Work out the finished part from the listing and answer in its coordinate system (mm). A direction names the side the tool comes from. Give positions to 0.01 mm unless a question says otherwise; leave off trailing zeros. Order: outer loops, then holes, each group sorted by start corner. A loop starts at its lowest first (then second) coordinate and runs counter-clockwise, first axis right, second up. Notation, with made-up numbers: (69, 39) - (106, 39) arc R18 cw to (106, 51) - close; hole circle Ø10 at (77.5, 59.5). An arc over 180 degrees is marked (long way). Return JSON: item names as keys, results as strings. Group by question number.
from build123d import *

# Parameters (mm, degrees)
SKETCH1_W                      = 57.15
SKETCH1_H                      = 32.639
BOSS_EXTRUDE1_DEPTH            = 0.762
F_3_0MM_DOWEL_HOLE1_D          = 3
SKETCH5_W                      = 4.5
SKETCH5_H                      = 5.9
BOSS_EXTRUDE2_DEPTH            = 6
SKETCH6_W                      = 3.23
SKETCH6_H                      = 4.63
CUT_EXTRUDE1_DEPTH             = 5.08
SKETCH7_R                      = 0.25
BOSS_EXTRUDE3_DEPTH            = 3.4
BOSS_EXTRUDE4_DEPTH            = 22.86
F_1_5MM_DOWEL_HOLE1_AT_2_COUNT = 2
F_1_5MM_DOWEL_HOLE1_AT_2_PITCH = 2.286
F_1_5MM_DOWEL_HOLE1_AT_3_COUNT = 2
F_1_5MM_DOWEL_HOLE1_AT_3_PITCH = 4.572
F_1_5MM_DOWEL_HOLE1_AT_4_COUNT = 2
F_1_5MM_DOWEL_HOLE1_AT_4_PITCH = 6.858
F_1_5MM_DOWEL_HOLE1_AT_5_COUNT = 2
F_1_5MM_DOWEL_HOLE1_AT_5_PITCH = 9.144
F_1_5MM_DOWEL_HOLE1_AT_6_COUNT = 2
F_1_5MM_DOWEL_HOLE1_AT_6_PITCH = 11.43
F_1_5MM_DOWEL_HOLE1_AT_7_COUNT = 2
F_1_5MM_DOWEL_HOLE1_AT_7_PITCH = 13.716
F_1_5MM_DOWEL_HOLE1_AT_8_COUNT = 2
F_1_5MM_DOWEL_HOLE1_AT_8_PITCH = 16.002
F_1_5MM_DOWEL_HOLE1_AT_9_COUNT = 2
F_1_5MM_DOWEL_HOLE1_AT_9_PITCH = 18.288
SKETCH13_W                     = 1.016
SKETCH13_H                     = 2.54
CUT_EXTRUDE2_DEPTH             = 1.27
LPATTERN1_COUNT                = 9
LPATTERN1_PITCH                = 2.286
MIRROR1_COPY_9_SKETCH_W        = 1.016
MIRROR1_COPY_9_SKETCH_H        = 2.54
MIRROR1_COPY_9_DEPTH           = 1.27
MIRROR1_COPY_10_SKETCH_W       = 1.016
MIRROR1_COPY_10_SKETCH_H       = 2.54
MIRROR1_COPY_10_DEPTH          = 1.27
MIRROR1_COPY_11_SKETCH_W       = 1.016
MIRROR1_COPY_11_SKETCH_H       = 2.54
MIRROR1_COPY_11_DEPTH          = 1.27
MIRROR1_COPY_12_SKETCH_W       = 1.016
MIRROR1_COPY_12_SKETCH_H       = 2.54
MIRROR1_COPY_12_DEPTH          = 1.27
MIRROR1_COPY_13_SKETCH_W       = 1.016
MIRROR1_COPY_13_SKETCH_H       = 2.54
MIRROR1_COPY_13_DEPTH          = 1.27
MIRROR1_COPY_14_SKETCH_W       = 1.016
MIRROR1_COPY_14_SKETCH_H       = 2.54
MIRROR1_COPY_14_DEPTH          = 1.27
MIRROR1_COPY_15_SKETCH_W       = 1.016
MIRROR1_COPY_15_SKETCH_H       = 2.54
MIRROR1_COPY_15_DEPTH          = 1.27
MIRROR1_COPY_16_SKETCH_W       = 1.016
MIRROR1_COPY_16_SKETCH_H       = 2.54
MIRROR1_COPY_16_DEPTH          = 1.27
SKETCH15_R                     = 5.715
BOSS_EXTRUDE5_DEPTH            = 9.652
SKETCH16_R                     = 1.905
CUT_EXTRUDE3_DEPTH             = 2.54


with BuildPart() as part:
    # Sketch1 → Boss-Extrude1 (new body)
    with BuildSketch(Plane(origin=(0, 0, 0), x_dir=(1, 0, 0), z_dir=(0, 1, 0))):
        Rectangle(SKETCH1_W, SKETCH1_H)
    extrude(amount=BOSS_EXTRUDE1_DEPTH)

    # Ø3.0mm Dowel Hole1 (through all)
    with Locations(Plane(origin=(0, 0.762, 0), x_dir=(1, 0, 0), z_dir=(0, 1, 0))):
        with Locations((-25.4, 13.1445), (-25.4, -13.1445), (25.4, -13.1445), (25.4, 13.1445)):
            Hole(F_3_0MM_DOWEL_HOLE1_D / 2)

    # Sketch5 → Boss-Extrude2 (add)
    with BuildSketch(Plane(origin=(0, 0.762, 0), x_dir=(1, 0, 0), z_dir=(0, 1, 0))):
        with Locations((-26.325, 0)):
            Rectangle(SKETCH5_W, SKETCH5_H)
    extrude(amount=BOSS_EXTRUDE2_DEPTH)

    # Sketch6 → Cut-Extrude1 (cut)
    with BuildSketch(Plane(origin=(0, 6.762, 0), x_dir=(1, 0, 0), z_dir=(0, 1, 0))):
        with Locations((-26.325, 0)):
            Rectangle(SKETCH6_W, SKETCH6_H)
    extrude(amount=-CUT_EXTRUDE1_DEPTH, mode=Mode.SUBTRACT)

    # Sketch7 → Boss-Extrude3 (add)
    with BuildSketch(Plane(origin=(0, 1.682, 0), x_dir=(1, 0, 0), z_dir=(0, 1, 0))):
        with Locations(Location((-26.875, 1, 0), (0, 0, 270))):
            Circle(SKETCH7_R)
        with Locations(Location((-26.875, -1, 0), (0, 0, 270))):
            Circle(SKETCH7_R)
    extrude(amount=BOSS_EXTRUDE3_DEPTH)

    # Sketch9 → Boss-Extrude4 (add)
    with BuildSketch(Plane(origin=(-24.075, 0, 0), x_dir=(0, 0, -1), z_dir=(1, 0, 0))):
        Polygon((0, 0), (0, 6.35), (2.54, 6.35), (3.926726593, 10.16), (7.736726593, 10.16), (8.89, 6.35), (8.89, 0), align=None)
    boss_extrude4 = extrude(amount=BOSS_EXTRUDE4_DEPTH)

    # Sketch11 → Ø1.5mm Dowel Hole1 (revolve, cut)
    with BuildSketch(Plane(origin=(-21.789, 10.16, -5.831726593), x_dir=(0, 0, 1), z_dir=(1, 0, 0))):
        Polygon((0, 0), (0, 0.704645464), (0.75, 0.254), (0.75, 0), align=None)
    f_1_5mm_dowel_hole1 = revolve(axis=Axis((-21.789, 16.51, -5.831726593), (0, -1, 0)), mode=Mode.SUBTRACT)

    # Ø1.5mm Dowel Hole1 at 2: Ø1.5mm Dowel Hole1 ×2
    with Locations(*[(i * F_1_5MM_DOWEL_HOLE1_AT_2_PITCH, 0, 0) for i in range(1, F_1_5MM_DOWEL_HOLE1_AT_2_COUNT)]):
        add(f_1_5mm_dowel_hole1, mode=Mode.SUBTRACT)

    # Ø1.5mm Dowel Hole1 at 3: Ø1.5mm Dowel Hole1 ×2
    with Locations(*[(i * F_1_5MM_DOWEL_HOLE1_AT_3_PITCH, 0, 0) for i in range(1, F_1_5MM_DOWEL_HOLE1_AT_3_COUNT)]):
        add(f_1_5mm_dowel_hole1, mode=Mode.SUBTRACT)

    # Ø1.5mm Dowel Hole1 at 4: Ø1.5mm Dowel Hole1 ×2
    with Locations(*[(i * F_1_5MM_DOWEL_HOLE1_AT_4_PITCH, 0, 0) for i in range(1, F_1_5MM_DOWEL_HOLE1_AT_4_COUNT)]):
        add(f_1_5mm_dowel_hole1, mode=Mode.SUBTRACT)

    # Ø1.5mm Dowel Hole1 at 5: Ø1.5mm Dowel Hole1 ×2
    with Locations(*[(i * F_1_5MM_DOWEL_HOLE1_AT_5_PITCH, 0, 0) for i in range(1, F_1_5MM_DOWEL_HOLE1_AT_5_COUNT)]):
        add(f_1_5mm_dowel_hole1, mode=Mode.SUBTRACT)

    # Ø1.5mm Dowel Hole1 at 6: Ø1.5mm Dowel Hole1 ×2
    with Locations(*[(i * F_1_5MM_DOWEL_HOLE1_AT_6_PITCH, 0, 0) for i in range(1, F_1_5MM_DOWEL_HOLE1_AT_6_COUNT)]):
        add(f_1_5mm_dowel_hole1, mode=Mode.SUBTRACT)

    # Ø1.5mm Dowel Hole1 at 7: Ø1.5mm Dowel Hole1 ×2
    with Locations(*[(i * F_1_5MM_DOWEL_HOLE1_AT_7_PITCH, 0, 0) for i in range(1, F_1_5MM_DOWEL_HOLE1_AT_7_COUNT)]):
        add(f_1_5mm_dowel_hole1, mode=Mode.SUBTRACT)

    # Ø1.5mm Dowel Hole1 at 8: Ø1.5mm Dowel Hole1 ×2
    with Locations(*[(i * F_1_5MM_DOWEL_HOLE1_AT_8_PITCH, 0, 0) for i in range(1, F_1_5MM_DOWEL_HOLE1_AT_8_COUNT)]):
        add(f_1_5mm_dowel_hole1, mode=Mode.SUBTRACT)

    # Ø1.5mm Dowel Hole1 at 9: Ø1.5mm Dowel Hole1 ×2
    with Locations(*[(i * F_1_5MM_DOWEL_HOLE1_AT_9_PITCH, 0, 0) for i in range(1, F_1_5MM_DOWEL_HOLE1_AT_9_COUNT)]):
        add(f_1_5mm_dowel_hole1, mode=Mode.SUBTRACT)

    # Sketch13 → Cut-Extrude2 (cut)
    with BuildSketch(Plane(origin=(0, 6.35, 0), x_dir=(1, 0, 0), z_dir=(0, 1, 0))):
        with Locations((-21.847835496, 1.27)):
            Rectangle(SKETCH13_W, SKETCH13_H)
    cut_extrude2 = extrude(amount=-CUT_EXTRUDE2_DEPTH, mode=Mode.SUBTRACT)

    # LPattern1: Cut-Extrude2 ×9
    with Locations(*[(i * LPATTERN1_PITCH, 0, 0) for i in range(1, LPATTERN1_COUNT)]):
        add(cut_extrude2, mode=Mode.SUBTRACT)

    # Mirror1: Boss-Extrude4, Ø1.5mm Dowel Hole1, Cut-Extrude2 across plane
    add(boss_extrude4.mirror(Plane.XY))
    add(f_1_5mm_dowel_hole1.mirror(Plane.XY), mode=Mode.SUBTRACT)
    add(cut_extrude2.mirror(Plane.XY), mode=Mode.SUBTRACT)

    # Mirror1 copy 1 sketch → Mirror1 copy 1 (revolve, cut)
    with BuildSketch(Plane(origin=(-19.503, 10.16, 5.831726593), x_dir=(0, 0, -1), z_dir=(1, 0, 0))):
        Polygon((0, 0), (0, -0.704645464), (0.75, -0.254), (0.75, 0), align=None)
    revolve(axis=Axis((-19.503, 16.51, 5.831726593), (0, 1, 0)), mode=Mode.SUBTRACT)

    # Mirror1 copy 2 sketch → Mirror1 copy 2 (revolve, cut)
    with BuildSketch(Plane(origin=(-17.217, 10.16, 5.831726593), x_dir=(0, 0, -1), z_dir=(1, 0, 0))):
        Polygon((0, 0), (0, -0.704645464), (0.75, -0.254), (0.75, 0), align=None)
    revolve(axis=Axis((-17.217, 16.51, 5.831726593), (0, 1, 0)), mode=Mode.SUBTRACT)

    # Mirror1 copy 3 sketch → Mirror1 copy 3 (revolve, cut)
    with BuildSketch(Plane(origin=(-14.931, 10.16, 5.831726593), x_dir=(0, 0, -1), z_dir=(1, 0, 0))):
        Polygon((0, 0), (0, -0.704645464), (0.75, -0.254), (0.75, 0), align=None)
    revolve(axis=Axis((-14.931, 16.51, 5.831726593), (0, 1, 0)), mode=Mode.SUBTRACT)

    # Mirror1 copy 4 sketch → Mirror1 copy 4 (revolve, cut)
    with BuildSketch(Plane(origin=(-12.645, 10.16, 5.831726593), x_dir=(0, 0, -1), z_dir=(1, 0, 0))):
        Polygon((0, 0), (0, -0.704645464), (0.75, -0.254), (0.75, 0), align=None)
    revolve(axis=Axis((-12.645, 16.51, 5.831726593), (0, 1, 0)), mode=Mode.SUBTRACT)

    # Mirror1 copy 5 sketch → Mirror1 copy 5 (revolve, cut)
    with BuildSketch(Plane(origin=(-10.359, 10.16, 5.831726593), x_dir=(0, 0, -1), z_dir=(1, 0, 0))):
        Polygon((0, 0), (0, -0.704645464), (0.75, -0.254), (0.75, 0), align=None)
    revolve(axis=Axis((-10.359, 16.51, 5.831726593), (0, 1, 0)), mode=Mode.SUBTRACT)

    # Mirror1 copy 6 sketch → Mirror1 copy 6 (revolve, cut)
    with BuildSketch(Plane(origin=(-8.073, 10.16, 5.831726593), x_dir=(0, 0, -1), z_dir=(1, 0, 0))):
        Polygon((0, 0), (0, -0.704645464), (0.75, -0.254), (0.75, 0), align=None)
    revolve(axis=Axis((-8.073, 16.51, 5.831726593), (0, 1, 0)), mode=Mode.SUBTRACT)

    # Mirror1 copy 7 sketch → Mirror1 copy 7 (revolve, cut)
    with BuildSketch(Plane(origin=(-5.787, 10.16, 5.831726593), x_dir=(0, 0, -1), z_dir=(1, 0, 0))):
        Polygon((0, 0), (0, -0.704645464), (0.75, -0.254), (0.75, 0), align=None)
    revolve(axis=Axis((-5.787, 16.51, 5.831726593), (0, 1, 0)), mode=Mode.SUBTRACT)

    # Mirror1 copy 8 sketch → Mirror1 copy 8 (revolve, cut)
    with BuildSketch(Plane(origin=(-3.501, 10.16, 5.831726593), x_dir=(0, 0, -1), z_dir=(1, 0, 0))):
        Polygon((0, 0), (0, -0.704645464), (0.75, -0.254), (0.75, 0), align=None)
    revolve(axis=Axis((-3.501, 16.51, 5.831726593), (0, 1, 0)), mode=Mode.SUBTRACT)

    # Mirror1 copy 9 sketch → Mirror1 copy 9 (cut)
    with BuildSketch(Plane(origin=(2.286, 6.35, 0), x_dir=(1, 0, 0), z_dir=(0, 1, 0))):
        with Locations((-21.847835496, -1.27)):
            Rectangle(MIRROR1_COPY_9_SKETCH_W, MIRROR1_COPY_9_SKETCH_H)
    extrude(amount=-MIRROR1_COPY_9_DEPTH, mode=Mode.SUBTRACT)

    # Mirror1 copy 10 sketch → Mirror1 copy 10 (cut)
    with BuildSketch(Plane(origin=(4.572, 6.35, 0), x_dir=(1, 0, 0), z_dir=(0, 1, 0))):
        with Locations((-21.847835496, -1.27)):
            Rectangle(MIRROR1_COPY_10_SKETCH_W, MIRROR1_COPY_10_SKETCH_H)
    extrude(amount=-MIRROR1_COPY_10_DEPTH, mode=Mode.SUBTRACT)

    # Mirror1 copy 11 sketch → Mirror1 copy 11 (cut)
    with BuildSketch(Plane(origin=(6.858, 6.35, 0), x_dir=(1, 0, 0), z_dir=(0, 1, 0))):
        with Locations((-21.847835496, -1.27)):
            Rectangle(MIRROR1_COPY_11_SKETCH_W, MIRROR1_COPY_11_SKETCH_H)
    extrude(amount=-MIRROR1_COPY_11_DEPTH, mode=Mode.SUBTRACT)

    # Mirror1 copy 12 sketch → Mirror1 copy 12 (cut)
    with BuildSketch(Plane(origin=(9.144, 6.35, 0), x_dir=(1, 0, 0), z_dir=(0, 1, 0))):
        with Locations((-21.847835496, -1.27)):
            Rectangle(MIRROR1_COPY_12_SKETCH_W, MIRROR1_COPY_12_SKETCH_H)
    extrude(amount=-MIRROR1_COPY_12_DEPTH, mode=Mode.SUBTRACT)

    # Mirror1 copy 13 sketch → Mirror1 copy 13 (cut)
    with BuildSketch(Plane(origin=(11.43, 6.35, 0), x_dir=(1, 0, 0), z_dir=(0, 1, 0))):
        with Locations((-21.847835496, -1.27)):
            Rectangle(MIRROR1_COPY_13_SKETCH_W, MIRROR1_COPY_13_SKETCH_H)
    extrude(amount=-MIRROR1_COPY_13_DEPTH, mode=Mode.SUBTRACT)

    # Mirror1 copy 14 sketch → Mirror1 copy 14 (cut)
    with BuildSketch(Plane(origin=(13.716, 6.35, 0), x_dir=(1, 0, 0), z_dir=(0, 1, 0))):
        with Locations((-21.847835496, -1.27)):
            Rectangle(MIRROR1_COPY_14_SKETCH_W, MIRROR1_COPY_14_SKETCH_H)
    extrude(amount=-MIRROR1_COPY_14_DEPTH, mode=Mode.SUBTRACT)

    # Mirror1 copy 15 sketch → Mirror1 copy 15 (cut)
    with BuildSketch(Plane(origin=(16.002, 6.35, 0), x_dir=(1, 0, 0), z_dir=(0, 1, 0))):
        with Locations((-21.847835496, -1.27)):
            Rectangle(MIRROR1_COPY_15_SKETCH_W, MIRROR1_COPY_15_SKETCH_H)
    extrude(amount=-MIRROR1_COPY_15_DEPTH, mode=Mode.SUBTRACT)

    # Mirror1 copy 16 sketch → Mirror1 copy 16 (cut)
    with BuildSketch(Plane(origin=(18.288, 6.35, 0), x_dir=(1, 0, 0), z_dir=(0, 1, 0))):
        with Locations((-21.847835496, -1.27)):
            Rectangle(MIRROR1_COPY_16_SKETCH_W, MIRROR1_COPY_16_SKETCH_H)
    extrude(amount=-MIRROR1_COPY_16_DEPTH, mode=Mode.SUBTRACT)

    # Sketch15 → Boss-Extrude5 (add)
    with BuildSketch(Plane(origin=(0, 0.762, 0), x_dir=(1, 0, 0), z_dir=(0, 1, 0))):
        with Locations(Location((5.135, 0, 0), (0, 0, 270))):
            Circle(SKETCH15_R)
    extrude(amount=BOSS_EXTRUDE5_DEPTH)

    # Sketch16 → Cut-Extrude3 (cut)
    with BuildSketch(Plane(origin=(0, 10.414, 0), x_dir=(1, 0, 0), z_dir=(0, 1, 0))):
        with Locations(Location((5.135, 0, 0), (0, 0, 270))):
            Circle(SKETCH16_R)
    extrude(amount=-CUT_EXTRUDE3_DEPTH, mode=Mode.SUBTRACT)


solid = part.part
1. The part is cut by section B-B (y = 4). Give the vertices of the cut face in (x, z) (3 decimals).
2. Consider probe 1 along Z at (x, y) = (25.4, 0.2); probe 2 along X at (y, z) = (2, 1.5) (3 decimals); probe 3 along Y at (x, z) = (18, -12). Determine where each line is inside the solid, lowest interval first. Write a range as from..to.
3. A tool of negligible diameter and unlimited length cuts with its end or side. For faces 1 (the flat face through (-26, 4, 2.95)), 2 (the flat face through (-3.6, 5.7, -2.54)), 3 (the cylindrical face through (-26.83, 0.38, -13.6)), from which of +Z, -Z, +X, -X, +Y, -Y can it reach the whole face along a straight path? Write none if from no direction.
4. Determine the mould class of faces 4 (the flat face through (-1.215, 4, 0)), 5 (the cylindrical face through (10.8, 5.52, -0.74)), 6 (the conical face through (-8.202, 9.534, -5.849)) for opening direction Z: released by +Z, released by -Z, zero draft, split by the parting line, or undercut.
5. Each of these flat-tipped pins is pushed along its axis until it touches: pin 1 (3 mm diameter, centred on y = 1.5, z = 9, fed in from +X) (3 decimals); pin 2 (1 mm diameter, centred on x = -19.5, z = 1.5, fed in from +Y); pin 3 (1.4 mm diameter, centred on x = -21.79, z = -5.83, fed in from +Y); pin 4 (3 mm diameter, centred on x = -7.5, z = 7, fed in from +Y). Where does it stop, or does it pass through?
6. The part is cut by section C-C (x = -25.4). State how many separate pieces and enclosed holes the cut face has, and give its area (3 significant figures).
7. The part is cut by section D-D (x = 15.5). Give the vertices of the cut face in (y, z), and give its area (3 significant figures).
8. The part is cut by section A-A (x = 25.4). Give the vertices of the cut face in (y, z).
Answers:
{
 "1": {"outline": "(-28.575, -2.95) - (-24.075, -2.95) - (-24.075, -8.89) - (-1.215, -8.89) - (-1.215, 8.89) - (-24.075, 8.89) - (-24.075, 2.95) - (-28.575, 2.95) - close; circle Ø0.5 at (-26.875, -1); circle Ø0.5 at (-26.875, 1); circle Ø11.43 at (5.135, 0); hole (-27.94, -2.315) - (-24.71, -2.315) - (-24.71, 2.315) - (-27.94, 2.315) - close"},
 "2": {"probe 1": "z = -16.32..-14.64, -11.64..11.64, 14.64..16.32", "probe 2": "x = -28.575..-27.94, -24.71..-1.215, -0.38..10.65", "probe 3": "y = 0..0.76"},
 "3": {"face 1": "+Z, -X, +Y", "face 2": "+Y", "face 3": "+Y, -Y"},
 "4": {"face 4": "zero draft", "face 5": "split by the parting line", "face 6": "undercut"},
 "5": {"pin 1": "stops at x = 28.575", "pin 2": "stops at y = 6.35", "pin 3": "stops at y = 9.88", "pin 4": "stops at y = 10.16"},
 "6": {"separate pieces": "3", "enclosed holes": "0", "area": "32.2 mm^2"},
 "7": {"outline": "(0, -16.32) - (0.76, -16.32) - (0.76, 16.32) - (0, 16.32) - close", "area": "24.9 mm^2"},
 "8": {"outline": "(0, -16.32) - (0.76, -16.32) - (0.76, -14.64) - (0, -14.64) - close; (0, -11.64) - (0.76, -11.64) - (0.76, 11.64) - (0, 11.64) - close; (0, 14.64) - (0.76, 14.64) - (0.76, 16.32) - (0, 16.32) - close"}
}
